```python
from build123d import *

# Parameters (mm, degrees)
SKETCH1_W                   = 56.235
SKETCH1_H                   = 16
SKETCH1_R                   = 2.35
SKETCH1_W_2                 = 2.5
SKETCH1_H_2                 = 12.2
BOSS_EXTRUDE1_DEPTH         = 3
ESQUISSE3_W                 = 22.7
ESQUISSE3_H                 = 11.84
ESQUISSE3_W_2               = 22.6
ENL_V_MAT_EXTRU_1_DEPTH     = 1
ESQUISSE4_R                 = 1
BOSS_EXTRU_2_DEPTH          = 3
R_VOLUTION1_ANGLE           = 90
R_VOLUTION1_OTHER_WAY_ANGLE = 90
ESQUISSE6_W                 = 2.5
ESQUISSE6_H                 = 16
BOSS_EXTRU_3_DEPTH          = 4.8
CONG_1_R                    = 2
CONG_2_R                    = 3
CONG_3_R                    = 1


with BuildPart() as part:
    # Sketch1 → Boss-Extrude1 (new body)
    with BuildSketch(Plane(origin=(0, 0, 0), x_dir=(1, 0, 0), z_dir=(0, 1, 0))):
        with Locations((28.1175, 8)):
            Rectangle(SKETCH1_W, SKETCH1_H)
        with Locations(Location((46.395, 8, 0), (0, 0, 270))):
            Circle(SKETCH1_R, mode=Mode.SUBTRACT)
        with Locations((7.685, 8)):
            Rectangle(SKETCH1_W_2, SKETCH1_H_2, mode=Mode.SUBTRACT)
    extrude(amount=BOSS_EXTRUDE1_DEPTH)

    # Esquisse3 → Enlèv. mat.-Extru.1 (cut)
    with BuildSketch(Plane.XZ):
        with Locations((11.35, -8)):
            Rectangle(ESQUISSE3_W, ESQUISSE3_H)
        with Locations((40.935, -8)):
            Rectangle(ESQUISSE3_W_2, ESQUISSE3_H)
    extrude(amount=-ENL_V_MAT_EXTRU_1_DEPTH, mode=Mode.SUBTRACT)

    # Esquisse4 → Boss.-Extru.2 (add)
    # profile 1 of 2: a face of its own
    with BuildSketch(Plane(origin=(0, 3, 0), x_dir=(1, 0, 0), z_dir=(0, 1, 0))):
        with BuildLine():
            Line((20.015, 16), (25.681747499, 20.374696879))
            ThreePointArc((25.681747499, 20.374696879), (27.515, 21), (29.348252501, 20.374696879))
            Line((29.348252501, 20.374696879), (35.015, 16))
            Line((35.015, 16), (27.515, 16))
            Line((27.515, 16), (20.015, 16))
        make_face()
        with Locations(Location((27.515, 18, 0), (0, 0, 270))):
            Circle(ESQUISSE4_R, mode=Mode.SUBTRACT)
    # profile 2 of 2: a face of its own
    with BuildSketch(Plane(origin=(0, 3, 0), x_dir=(1, 0, 0), z_dir=(0, 1, 0))):
        with BuildLine():
            Line((27.515, 0), (35.015, 0))
            Line((35.015, 0), (29.348252501, -4.374696879))
            ThreePointArc((29.348252501, -4.374696879), (27.515, -5), (25.681747499, -4.374696879))
            Line((25.681747499, -4.374696879), (20.015, 0))
            Line((20.015, 0), (27.515, 0))
        make_face()
        with Locations(Location((27.515, -2, 0), (0, 0, 90))):
            Circle(ESQUISSE4_R, mode=Mode.SUBTRACT)
    extrude(amount=-BOSS_EXTRU_2_DEPTH)



with BuildPart() as body_2:
    # Esquisse5 → Révolution1 (revolve)
    with BuildSketch(Plane.XY.offset(-8)):
        Polygon((-2.25, 0.84), (2.5, 0.84), (2.5, -1.66), (0.25, -1.66), (0.25, -4.86), (-2.25, -4.86), align=None)
    revolve(axis=Axis((-14.237579535, -15.86, -8), (-1, 0, 0)), revolution_arc=R_VOLUTION1_ANGLE)

    # Esquisse5 → Révolution1 other way (revolve)
    with BuildSketch(Plane.XY.offset(-8)):
        Polygon((-2.25, 0.84), (2.5, 0.84), (2.5, -1.66), (0.25, -1.66), (0.25, -4.86), (-2.25, -4.86), align=None)
    revolve(axis=Axis((-14.237579535, -15.86, -8), (1, 0, 0)), revolution_arc=R_VOLUTION1_OTHER_WAY_ANGLE)


with BuildPart() as part_1:
    add(part.part)

    add(body_2.part)  # Boss.-Extru.3 merges body 2
    # Esquisse6 → Boss.-Extru.3 (add)
    with BuildSketch(Plane(origin=(0, 3, 0), x_dir=(1, 0, 0), z_dir=(0, 1, 0))):
        with Locations((1.25, 8)):
            Rectangle(ESQUISSE6_W, ESQUISSE6_H)
    extrude(amount=-BOSS_EXTRU_3_DEPTH)

    # Congé1
    cong_1_edges = [part_1.edges().sort_by_distance(p)[0] for p in [
        (0, 3, -8),
    ]]
    fillet(cong_1_edges, radius=CONG_1_R)

    # Congé2
    cong_2_edges = [part_1.edges().sort_by_distance(p)[0] for p in [
        (56.235, 1.5, -16),
        (56.235, 1.5, 0),
    ]]
    fillet(cong_2_edges, radius=CONG_2_R)

    # Congé3
    cong_3_edges = [part_1.edges().sort_by_distance(p)[0] for p in [
        (-2.25, 0.84, -8),
    ]]
    fillet(cong_3_edges, radius=CONG_3_R)


solid = part_1.part
```
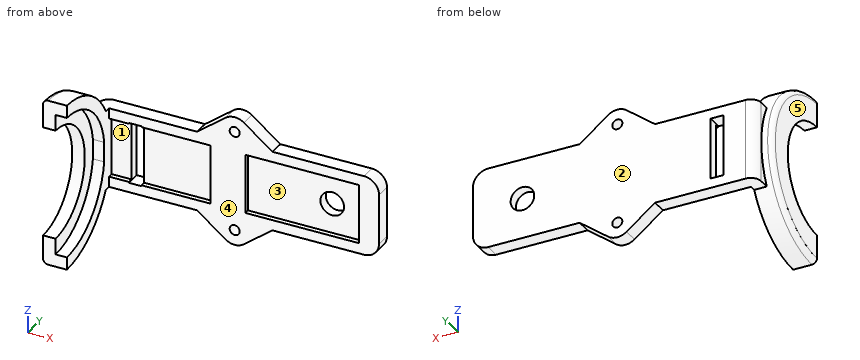
Geometry check sheet. Reference: the model listing, model coordinates, mm. Face numbers are marked on the shaded views. A direction names the side the tool comes from. Round coordinates to 2 decimals unless told otherwise and drop trailing zeros. Order: outer loops, then holes, each group sorted by start corner. A loop starts at its lowest first (then second) coordinate and runs counter-clockwise, first axis right, second up. Notation, with made-up numbers: (31.5, -36.5) - (61.5, -36.5) arc R33 ccw to (61.5, -6.5) - close; hole circle Ø9 at (-24, 50.25). An arc over 180 degrees is marked (long way). Use a Markdown table: item, result. Add a question column.
(1) Depth check by flat-ended pin: pin 1 (0.5 mm diameter, centred on x = 19, y = 0.5, fed in from -Z); pin 2 (0.8 mm diameter, centred on y = 0.5, z = -6, fed in from -X); pin 3 (1.2 mm diameter, centred on x = 5, z = -5.5, fed in from -Y). Enter the tip coordinate at first touch or a pass-through.
(2) Sectioned sample at B-B, the plane x = 43. Enter the section's corners in (y, z).
(3) Tool access check on the marked faces 1 and 2. Record the directions out of +Z, -Z, +X, -X, +Y, -Y that give a thin tool (end or side, any length) a straight path to the whole face; none if there is none.
(4) Sectioned sample at A-A, the plane z = -8. Enter the section's corners in (x, y) (3 decimals).
(5) Release check for a two-part mould opening along X. For the marked faces 3, 4 and 5 record: pulls with the +X half, pulls with the -X half, needs draft (parallel to the pull), parting line crosses it, or undercut.
(6) Material ranges on line 1 along Y through (x, z) = (34, -9); line 2 along X through (y, z) = (1.45, -8) (3 decimals); line 3 along Y through (x, z) = (27.5, -11.5), recorded low to high. Write a range as [from, to].
(7) Sectioned sample at C-C, the plane z = 2. Count the separate pieces of the cut face and the enclosed holes in it, and give its area (3 significant figures).
Answers below:
| question | item | result |
|---|---|---|
| 1 | pin 1 | z = -16 |
| 1 | pin 2 | x = -2.17 |
| 1 | pin 3 | y = 1 |
| 2 | outline | (0, -16) - (3, -16) - (3, 0) - (0, 0) - (0, -2.08) - (1, -2.08) - (1, -13.92) - (0, -13.92) - close |
| 3 | face 1 | -Y |
| 3 | face 2 | +Z, -Z, +X, -X, +Y |
| 4 | outline | (-2.25, -4.86) - (0.25, -4.86) - (0.25, -1.8) - (2.5, -1.8) - (2.5, 1) - (6.435, 1) - (6.435, 3) - (2, 3) arc R2 ccw to (0, 1) - (0, 0.84) - (-1.25, 0.84) arc R1 ccw to (-2.25, -0.16) - close; (8.935, 1) - (22.7, 1) - (22.7, 0) - (29.635, 0) - (29.635, 1) - (44.045, 1) - (44.045, 3) - (8.935, 3) - close; (48.745, 1) - (52.235, 1) - (52.235, 0) - (56.235, 0) - (56.235, 3) - (48.745, 3) - close |
| 5 | face 3 | undercut |
| 5 | face 4 | needs draft |
| 5 | face 5 | pulls with the -X half |
| 6 | line 1 | [1, 3] |
| 6 | line 2 | [0.051, 6.435], [8.935, 44.045], [48.745, 56.235] |
| 6 | line 3 | [0, 3] |
| 7 | separate pieces | 3 |
| 7 | enclosed holes | 0 |
| 7 | area | 52.6 mm² |
